Verification items for the finished model (mm, model axes). Face numbers are marked on the shaded views. A direction names the side the tool comes from. Round coordinates to 2 decimals unless told otherwise and drop trailing zeros. Order: outer loops, then holes, each group sorted by start corner. A loop starts at its lowest first (then second) coordinate and runs counter-clockwise, first axis right, second up. Notation, with made-up numbers: M -31,8.5 L 16,8.5 A18 cw 16,16.5 Z; hole C 62,80.25 d4. An arc over 180 degrees is marked long. Answer as a JSON object with one key per item and string values. Group by question number.
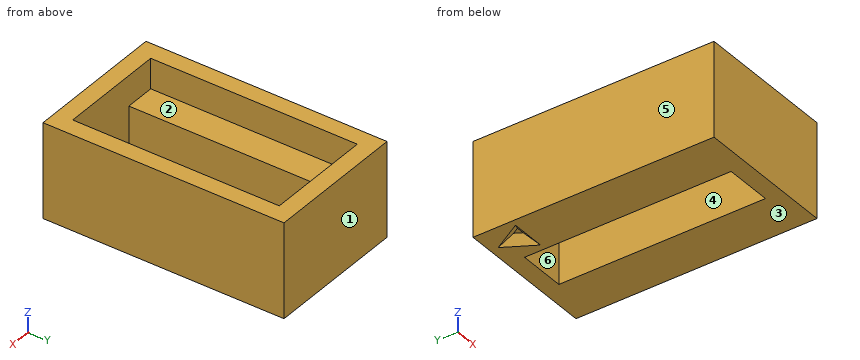
```python
from build123d import *

# Parameters (mm, degrees)
BOX014_W                   = 5.5
BOX014_H                   = 24
BOX014_DEPTH               = 8
BOX016_W                   = 12.5
BOX016_H                   = 24
BOX016_DEPTH               = 4
PAD009_DEPTH               = 1.1
CHAMFER001_SIZE            = 1
CHAMFER001_PLACEMENT_ANGLE = 180
BOX015_W                   = 16.5
BOX015_H                   = 28
BOX015_DEPTH               = 11


with BuildPart() as cube014:
    # Box014 → Box014 (new body)
    with BuildSketch(Plane(origin=(3.25, -9, -0.5), x_dir=(1, 0, 0), z_dir=(0, 0, 1))):
        with Locations((2.75, 12)):
            Rectangle(BOX014_W, BOX014_H)
    extrude(amount=BOX014_DEPTH)


with BuildPart() as cube016:
    # Box016 → Box016 (new body)
    with BuildSketch(Plane(origin=(-0.25, -9, 7.5), x_dir=(1, 0, 0), z_dir=(0, 0, 1))):
        with Locations((6.25, 12)):
            Rectangle(BOX016_W, BOX016_H)
    extrude(amount=BOX016_DEPTH)


with BuildPart() as fusion010:
    # Sketch012 → Pad009 (new body)
    with BuildSketch(Plane.XY):
        Polygon((0, 20.777284), (-2.180816, 17), (2.180816, 17), align=None)
    extrude(amount=PAD009_DEPTH)

    # Chamfer001
    chamfer001_edges = [fusion010.edges().sort_by_distance(p)[0] for p in [
        (-1.090408, 18.888642, 0),
        (0, 17, 0),
        (1.090408, 18.888642, 0),
    ]]
    chamfer(chamfer001_edges, length=CHAMFER001_SIZE)


with BuildPart() as fusion010_1:
    # Chamfer001 placement: moved
    add(fusion010.part.moved(Location((0.5, -4.5, 0.9))).rotate(Axis((0.5, -4.5, 0.9), (0, 1, 0)), CHAMFER001_PLACEMENT_ANGLE))

    # Fusion010: union Cube014, Cube016
    add(cube014.part)
    add(cube016.part)


with BuildPart() as obj1:
    # Box015 → Box015 (new body)
    with BuildSketch(Plane(origin=(-2.25, -11, 0), x_dir=(1, 0, 0), z_dir=(0, 0, 1))):
        with Locations((8.25, 14)):
            Rectangle(BOX015_W, BOX015_H)
    extrude(amount=BOX015_DEPTH)

    # Cut021: cut Fusion010
    add(fusion010_1.part, mode=Mode.SUBTRACT)


solid = obj1.part
```
Q1. Cross-section at A-A, the plane y = -8.25. Record the cut outline in (x, z).
Q2. Release check for a two-part mould opening along Y. For the marked faces 1, 2 and 3 record: released by +Y, released by -Y, zero draft, split by the parting line, or undercut.
Q3. Thickness scan on line 1 (Y direction, x = 0.75, z = 9); line 2 (X direction, y = -5, z = 2); line 3 (X direction, y = -8.5, z = 10.25). Record the ranges inside material, lowest first. Write a range as from..to.
Q4. Cross-section at B-B, the plane x = 8.25. Record the cut outline in (y, z), then the cut area to 3 significant figures.
Q5. Cross-section at C-C, the plane z = 1.5. Record the cut outline in (x, y), then the cut area to 3 significant figures.
Q6. Gauge pin test, flat end, axial feed: pin 1 Ø3 at (x, y) = (2, 5) entering from +Z. Record the tip position at first contact, or that the pin passes through.
Q7. Tool access check on the marked faces 4, 5 and 6. Record the directions out of +Z, -Z, +X, -X, +Y, -Y that give a thin tool (end or side, any length) a straight path to the whole face; none if there is none.
Conclusion:
{
 "1": {"outline": "M -2.25,0 L 3.25,0 L 3.25,7.5 L -0.25,7.5 L -0.25,11 L -2.25,11 Z; M 8.75,0 L 14.25,0 L 14.25,11 L 12.25,11 L 12.25,7.5 L 8.75,7.5 Z"},
 "2": {"face 1": "released by +Y", "face 2": "undercut", "face 3": "zero draft"},
 "3": {"line 1": "-11..-9, 15..17", "line 2": "-2.25..3.25, 8.75..14.25", "line 3": "-2.25..-0.25, 12.25..14.25"},
 "4": {"outline": "M -11,0 L -9,0 L -9,11 L -11,11 Z; M 15,0 L 17,0 L 17,11 L 15,11 Z", "area": "44.0 mm2"},
 "5": {"outline": "M -2.25,-11 L 14.25,-11 L 14.25,17 L -2.25,17 Z; hole M 3.25,-9 L 8.75,-9 L 8.75,15 L 3.25,15 Z", "area": "330 mm2"},
 "6": {"pin 1": "z = 7.5"},
 "7": {"face 4": "+Z, -Z", "face 5": "+Z, -Z, -X, +Y, -Y", "face 6": "+Z"}
}
